Input: part model. Units: mm. Frame: model coordinates. A direction names the side the tool comes from. Coordinates: 2 decimals unless noted, no trailing zeros. Loops run counter-clockwise (first coordinate to the right, second up) from the corner with the lowest first, then second, coordinate; pieces in that order, holes last. Notation, with made-up numbers: (69.25, 7.5) -> (111.25, 7.5) arc R11 ccw to (111.25, 24.5) -> close; hole circle Ø11 at (-39.75, 25.25). An arc over 180 degrees is marked (long way). Answer as a JSON object with one key per item and string values.
from build123d import *

# Parameters (mm, degrees)
F0_W     = 19.304
F0_H     = 19.304
F1_DEPTH = 6.35
F2_W     = 19.304
F2_H     = 19.304
F2_R     = 2.54
F3_DEPTH = 3.175
F4_R     = 2.54
F5_DEPTH = 3.175


with BuildPart() as f1:
    # F0 (on Top) → F1 (new body)
    with BuildSketch(Plane.XY):
        Rectangle(F0_W, F0_H)
    extrude(amount=F1_DEPTH)

    # F2 (on face) → F3 (cut)
    with BuildSketch(Plane.XY.offset(6.35)):
        Rectangle(F2_W, F2_H)
        with Locations((0, -5.08)):
            Circle(F2_R, mode=Mode.SUBTRACT)
        with Locations((0, 5.08)):
            Circle(F2_R, mode=Mode.SUBTRACT)
    extrude(amount=-F3_DEPTH, mode=Mode.SUBTRACT)

    # F4 (on face) → F5 (cut)
    with BuildSketch(Plane.XY.offset(3.175)):
        with Locations((5.08, 0)):
            Circle(F4_R)
        with Locations((-5.08, 0)):
            Circle(F4_R)
    extrude(amount=-F5_DEPTH, mode=Mode.SUBTRACT)


solid = f1.part
1. Line query: line 1 along Y through (x, z) = (5.08, 2); line 2 along X through (y, z) = (-2, 1.25); line 3 along X through (y, z) = (-1, 1.5). Output: solid intervals per line, ascending.
Reply:
{"line 1": "y = -9.65 to -2.54, 2.54 to 9.65", "line 2": "x = -9.65 to -6.65, -3.51 to 3.51, 6.65 to 9.65", "line 3": "x = -9.65 to -7.41, -2.75 to 2.75, 7.41 to 9.65"}
2. Section query D-D (y = -5.08). Return loops of the section in (x, z) (3 decimals), plus the area to 3 significant figures.
Reply:
{"outline": "(-9.652, 0) -> (9.652, 0) -> (9.652, 3.175) -> (2.54, 3.175) -> (2.54, 6.35) -> (-2.54, 6.35) -> (-2.54, 3.175) -> (-9.652, 3.175) -> close", "area": "77.4 mm2"}
3. Section query B-B (z = 2.75). Return loops of the section in (x, y), plus the area to 3 significant figures.
Reply:
{"outline": "(-9.65, -9.65) -> (9.65, -9.65) -> (9.65, 9.65) -> (-9.65, 9.65) -> close; hole circle Ø5.08 at (-5.08, 0); hole circle Ø5.08 at (5.08, 0)", "area": "332 mm2"}
4. Pin query (flat end, axial travel): P1, Ø3, axis at x = 7.5, y = 4, coming from the +Z side (3 decimals). Return the tip coordinate at first contact, or that it passes through.
Reply:
{"P1": "stops at z = 3.175"}
5. Section query C-C (x = 0). Return loops of the section in (y, z) (3 decimals), plus the area to 3 significant figures.
Reply:
{"outline": "(-9.652, 0) -> (9.652, 0) -> (9.652, 3.175) -> (7.62, 3.175) -> (7.62, 6.35) -> (2.54, 6.35) -> (2.54, 3.175) -> (-2.54, 3.175) -> (-2.54, 6.35) -> (-7.62, 6.35) -> (-7.62, 3.175) -> (-9.652, 3.175) -> close", "area": "93.5 mm2"}
6. Access query for faces 4 (the face through (0, 0, 3.175)), 5 (the face through (0, 5, 6.35)). Directions: +Z, -Z, +X, -X, +Y, -Y. A direction counts if a zero-diameter tool reaches every point of the face in a straight line with its end or side. Return the directions, or none.
Reply:
{"face 4": "+Z", "face 5": "+Z, +X, -X, +Y, -Y"}
7. Mould query, pull axis Y, two halves, no side actions, for faces 1 (the face through (-0.55, 2.6, 4.78)), 2 (the face through (0, -9.652, 2)), 3 (the face through (0, -5, 6.35)). Classes: pulls with the +Y half, pulls with the -Y half, needs draft (parallel to the pull), parting line crosses it, or undercut.
Reply:
{"face 1": "undercut", "face 2": "pulls with the -Y half", "face 3": "needs draft"}
8. Section query A-A (x = 5.08). Return loops of the section in (y, z) (3 decimals).
Reply:
{"outline": "(-9.652, 0) -> (-2.54, 0) -> (-2.54, 3.175) -> (-9.652, 3.175) -> close; (2.54, 0) -> (9.652, 0) -> (9.652, 3.175) -> (2.54, 3.175) -> close"}
